Autodesk Inventor part; units mm, degrees
ref_plane "Start Plane" through (0, 0, 0) normal (0, 0, 1) x (1, 0, 0)
ref_plane "End Plane" through (0, 0, 762) normal (0, 0, 1) x (1, 0, 0)
ref_plane "Work Plane5" through (-895.35, -25.4, 762) normal (-1, 0, 0) x (0, 0, 1)
ref_plane "Start Plane" through (0, 0, 0) normal (0, 0, 1) x (1, 0, 0)
ref_plane "End Plane" through (0, 0, 762) normal (0, 0, 1) x (1, 0, 0)
sketch "Sketch" plane through (0, 0, 0) normal (0, 0, 1) x (1, 0, 0)
  line L0 (-19.05, 19.05) -> (19.05, 19.05)
  line L1 (19.05, 19.05) -> (19.05, -19.05)
  line L2 (19.05, -19.05) -> (-19.05, -19.05)
  line L3 (-19.05, -19.05) -> (-19.05, 19.05)
  line L4 (15.875, 15.875) -> (-15.875, 15.875)
  line L5 (-15.875, 15.875) -> (-15.875, -15.875)
  line L6 (-15.875, -15.875) -> (15.875, -15.875)
  line L7 (15.875, -15.875) -> (15.875, 15.875)
  point P0 (0, 0)
  point P1 (0, 19.05)
  point P2 (-19.05, 0)
  dimension "width" = 38.1
  dimension "d1" = 3.175
extrude "Body" add sketch "Sketch" along normal up to surface (762 mm away) from surface at 0
sketch "Sketch4" plane through (0, 0, 0) normal (0, 0, 1) x (1, 0, 0)
  line L0 (0, 0) -> (10, 0)
ref_plane "Work Plane4" through (0, 0, 0) normal (0, -1, 0) x (1, 0, 0)
sketch "Sketch5" plane through (0, 0, 0) normal (0, -1, 0) x (1, 0, 0)
  line L0 (-2, 0) -> (12, 0)
  line L1 (-2, 762) -> (12, 762)
  dimension "d9" = 762
ref_plane "Work Plane5" through (-895.35, -25.4, 762) normal (-1, 0, 0) x (0, 0, 1)
ref_plane "Work Plane6" through (234.95, -25.4, 0) normal (1, 0, 0) x (0, 0, -1)
ref_plane "Work Plane7" through (-330.2, -6.35, 6.35) normal (1, 0, 0) x (0, 0, -1)
sketch "Sketch6" plane through (-330.2, -6.35, 6.35) normal (1, 0, 0) x (0, 0, -1)
  line L0 (-25.4, 12.7) -> (25.4, 12.7)
  line L1 (25.4, 12.7) -> (25.4, -12.7)
  line L2 (25.4, -12.7) -> (-25.4, -12.7)
  line L3 (-25.4, -12.7) -> (-25.4, 12.7)
  line L4 (22.225, 9.525) -> (-22.225, 9.525)
  line L5 (-22.225, 9.525) -> (-22.225, -9.525)
  line L6 (-22.225, -9.525) -> (22.225, -9.525)
  line L7 (22.225, -9.525) -> (22.225, 9.525)
extrude "Extrusion3" cut sketch "Sketch6" along normal up to surface (1130.3 mm away) from surface at -565.15 contours L0 L1 L2 L3 | L7 L6 L5 L4
ref_plane "Work Plane8" through (-895.35, -25.4, 762) normal (-1, 0, 0) x (0, 0, 1)
ref_plane "Work Plane9" through (234.95, -25.4, 0) normal (1, 0, 0) x (0, 0, -1)
ref_plane "Work Plane10" through (-330.2, -6.35, 755.65) normal (1, 0, 0) x (0, 0, -1)
sketch "Sketch7" plane through (-330.2, -6.35, 755.65) normal (1, 0, 0) x (0, 0, -1)
  line L0 (-25.4, 12.7) -> (25.4, 12.7)
  line L1 (25.4, 12.7) -> (25.4, -12.7)
  line L2 (25.4, -12.7) -> (-25.4, -12.7)
  line L3 (-25.4, -12.7) -> (-25.4, 12.7)
  line L4 (22.225, 9.525) -> (-22.225, 9.525)
  line L5 (-22.225, 9.525) -> (-22.225, -9.525)
  line L6 (-22.225, -9.525) -> (22.225, -9.525)
  line L7 (22.225, -9.525) -> (22.225, 9.525)
extrude "Extrusion4" cut sketch "Sketch7" along normal up to surface (1130.3 mm away) from surface at -565.15 contours L0 L1 L2 L3 | L7 L6 L5 L4
equation "\"G_OFFSET_START\" = 0"
equation "\"G_OFFSET_END\" = 0"
equation "\"d5\" = length + G_OFFSET_END"
equation "\"G_L\" = 762"
properties part number "1.5x1.5x.125 Tube" material "Aluminum-6061"
Verification items for the finished model (mm, model axes). A direction names the side the tool comes from. Give positions to 0.01 mm unless a question says otherwise; leave off trailing zeros. Order: outer loops, then holes, each group sorted by start corner. A loop starts at its lowest first (then second) coordinate and runs counter-clockwise, first axis right, second up. Notation, with made-up numbers: (75.5, 36.25) -> (120.5, 36.25) arc R4 ccw to (120.5, 43.25) -> close; hole circle Ø4 at (-7.75, -30). An arc over 180 degrees is marked (long way). Use a Markdown table: item, result.
1) Mould release check, pull along Y, two halves, no side actions. Record for faces 1 (the flat face through (0, -19.05, 376)), 2 (the flat face through (0, 19.05, 376)), 3 (the flat face through (15.875, 0, 376)), 4 (the flat face through (19.05, 0, 376)): pulls with the +Y half, pulls with the -Y half, needs draft (parallel to the pull), parting line crosses it, or undercut.
Results:
| item | result |
|---|---|
| face 1 | pulls with the -Y half |
| face 2 | pulls with the +Y half |
| face 3 | undercut |
| face 4 | needs draft |
2) Section check B-B, the plane y = -2. Record the boundary of the cut face in (x, z) (3 decimals), then the cut area to 3 significant figures.
Results:
| item | result |
|---|---|
| outline | (-19.05, 31.75) -> (-15.875, 31.75) -> (-15.875, 730.25) -> (-19.05, 730.25) -> close; (15.875, 31.75) -> (19.05, 31.75) -> (19.05, 730.25) -> (15.875, 730.25) -> close |
| area | 4,440 mm² |
3) Tool access check on faces 5 (the flat face through (-15.875, 0, 376)), 6 (the flat face through (-2, -17, 730.25)), 7 (the flat face through (0, 17, 0)), 8 (the flat face through (0, -17, 31.75)), 9 (the flat face through (0, 17, 762)). Record the directions out of +Z, -Z, +X, -X, +Y, -Y that give a thin tool (end or side, any length) a straight path to the whole face; none if there is none.
Results:
| item | result |
|---|---|
| face 5 | +Z, -Z |
| face 6 | +Z, +X, -X, -Y |
| face 7 | -Z, +X, -X, +Y, -Y |
| face 8 | -Z, +X, -X, -Y |
| face 9 | +Z, +X, -X, +Y, -Y |
4) Depth check by flat-ended pin: pin 1 Ø2.5 at (x, z) = (17, 741) entering from -Y; pin 2 Ø7.5 at (x, y) = (3.5, -9.5) entering from +Z. Enter the tip coordinate at first touch or a pass-through.
Results:
| item | result |
|---|---|
| pin 1 | y = 6.35 |
| pin 2 | through |
5) Material ranges on probe 1 along Y at (x, z) = (10, 622) (3 decimals); probe 2 along Z at (x, y) = (-16, -14), recorded low to high.
Results:
| item | result |
|---|---|
| probe 1 | -19.05 to -15.875, 15.875 to 19.05 |
| probe 2 | 31.75 to 730.25 |
6) Section check A-A, the plane x = -1. Record the boundary of the cut face in (y, z) (3 decimals).
Results:
| item | result |
|---|---|
| outline | (-19.05, 31.75) -> (-15.875, 31.75) -> (-15.875, 730.25) -> (-19.05, 730.25) -> close; (15.875, 0) -> (19.05, 0) -> (19.05, 762) -> (15.875, 762) -> close |
7) Section check C-C, the plane z = 310. Record the boundary of the cut face in (x, y) (3 decimals), then the cut area to 3 significant figures.
Results:
| item | result |
|---|---|
| outline | (-19.05, -19.05) -> (19.05, -19.05) -> (19.05, 19.05) -> (-19.05, 19.05) -> close; hole (-15.875, -15.875) -> (15.875, -15.875) -> (15.875, 15.875) -> (-15.875, 15.875) -> close |
| area | 444 mm² |
